Build history of the part. All positions in model axes, mm. A direction names the side the tool comes from. Round coordinates to 2 decimals unless told otherwise and drop trailing zeros. Write each loop counter-clockwise with the first axis right and the second up, starting at its lowest first coordinate (ties: lowest second). Pieces come first, ordered by that corner, then holes. Notation, with made-up numbers: (4, 37.25) -> (17, 37.25) arc R32 ccw to (17, 72.25) -> close; hole circle Ø7 at (36.25, 58.5). An arc over 180 degrees is marked (long way). Answer in a Markdown table with one row per item. Add a question column.
from build123d import *

# Parameters (mm, degrees)
SKETCH_W     = 44
SKETCH_H     = 46
PAD_DEPTH    = 7
SKETCH001_W  = 25.8
SKETCH001_H  = 25.8
POCKET_DEPTH = 8
SKETCH002_W  = 6.75
SKETCH002_H  = 3
PAD001_DEPTH = 50
SKETCH006_W  = 6.75
SKETCH006_H  = 4.5
PAD017_DEPTH = 9


with BuildPart() as part:
    # Sketch → Pad (new body)
    with BuildSketch(Plane.XY):
        with Locations((-22, -23)):
            Rectangle(SKETCH_W, SKETCH_H)
    extrude(amount=PAD_DEPTH)

    # Sketch001 (on Face6 of Pad) → Pocket (cut)
    with BuildSketch(Plane.XY.offset(7)):
        with Locations((-22, -24.9)):
            Rectangle(SKETCH001_W, SKETCH001_H)
    extrude(amount=-POCKET_DEPTH, mode=Mode.SUBTRACT)

    # Sketch002 (on Face5 of Pocket) → Pad001 (new body)
    with BuildSketch(Plane.XY.offset(7)):
        with Locations((-40.625, -10.5)):
            Rectangle(SKETCH002_W, SKETCH002_H)
    extrude(amount=PAD001_DEPTH)

    # Sketch006 (on Face14 of Pad001) → Pad017 (new body)
    with BuildSketch(Plane(origin=(0, -9, 0), x_dir=(-1, 0, 0), z_dir=(0, 1, 0))):
        with Locations((40.625, 54.75)):
            Rectangle(SKETCH006_W, SKETCH006_H)
    extrude(amount=PAD017_DEPTH)


solid = part.part
(1) Which spindle directions (+Z, -Z, +X, -X, +Y, -Y) get a long thin tool onto all of the face, cutting with end or side? Do faces 1 (the face through (-22, -37.8, 4)), 2 (the face through (-37.25, -10, 36)), 3 (the face through (-41, -12, 32)). Say none if no direction does.
(2) Drop flat-ended pins along their axis: P1, Ø10, axis at y = -8.5, z = 25.5, coming from the +X side; P2, Ø3.5, axis at x = -21, z = 5, coming from the +Y side; P3, Ø5.5, axis at x = -39.5, z = 19, coming from the +Y side; P4, Ø2, axis at x = -11, y = -38, coming from the +Z side. Give the stop position or say it passes through.
(3) Saw through at B-B (y = -21). List the corners of the cut face in (x, z).
(4) Saw through at A-A (x = -21.5). List the corners of the cut face in (y, z).
(5) Saw through at D-D (x = -39.5). List the corners of the cut face in (y, z), plus the area to 4 significant figures.
(6) Mould opens along Z. For faces 4 (the face through (-41, -5, 52.5)), 5 (the face through (-34.9, -25, 4)), 6 (the face through (-41, -9, 29)), 7 (the face through (-8, -23, 0)) say: pulls with the +Z half, pulls with the -Z half, needs draft (parallel to the pull), parting line crosses it, or undercut.
(7) Probe line 1 along Z through (x, y) = (-4, -39); line 2 along X through (y, z) = (-10.5, 24.5); line 3 along Y through (x, z) = (-38, 51). List the from-to ranges inside material, lowest first.
(8) Saw through at C-C (y = -11). List the corners of the cut face in (x, z).
Answer sheet:
| question | item | result |
|---|---|---|
| 1 | face 1 | +Z, -Z |
| 1 | face 2 | +Z, +X, +Y, -Y |
| 1 | face 3 | +Z, +X, -X, -Y |
| 2 | P1 | stops at x = -37.25 |
| 2 | P2 | stops at y = 0 |
| 2 | P3 | stops at y = -9 |
| 2 | P4 | stops at z = 7 |
| 3 | outline | (-44, 0) -> (-34.9, 0) -> (-34.9, 7) -> (-44, 7) -> close; (-9.1, 0) -> (0, 0) -> (0, 7) -> (-9.1, 7) -> close |
| 4 | outline | (-46, 0) -> (-37.8, 0) -> (-37.8, 7) -> (-46, 7) -> close; (-12, 0) -> (0, 0) -> (0, 7) -> (-12, 7) -> close |
| 5 | outline | (-46, 0) -> (0, 0) -> (0, 7) -> (-9, 7) -> (-9, 52.5) -> (0, 52.5) -> (0, 57) -> (-12, 57) -> (-12, 7) -> (-46, 7) -> close |
| 5 | area | 512.5 mm² |
| 6 | face 4 | undercut |
| 6 | face 5 | needs draft |
| 6 | face 6 | undercut |
| 6 | face 7 | pulls with the -Z half |
| 7 | line 1 | z = 0 to 7 |
| 7 | line 2 | x = -44 to -37.25 |
| 7 | line 3 | y = -12 to -9 |
| 8 | outline | (-44, 0) -> (0, 0) -> (0, 7) -> (-37.25, 7) -> (-37.25, 57) -> (-44, 57) -> close |
